Study the drawing (mm; zero at the part's minimum x, y, z) and answer. Coordinates: 2 decimals unless noted, no trailing zeros. Loops run counter-clockwise (first coordinate to the right, second up) from the corner with the lowest first, then second, coordinate; pieces in that order, holes last. Notation, with made-up numbers: (51.5, -30.5) -> (69.5, -30.5) arc R22 ccw to (69.5, -4.5) -> close; hole circle Ø10 at (35.25, 76.5). An arc over 180 degrees is marked (long way). One line per question, with ' | ' between items.
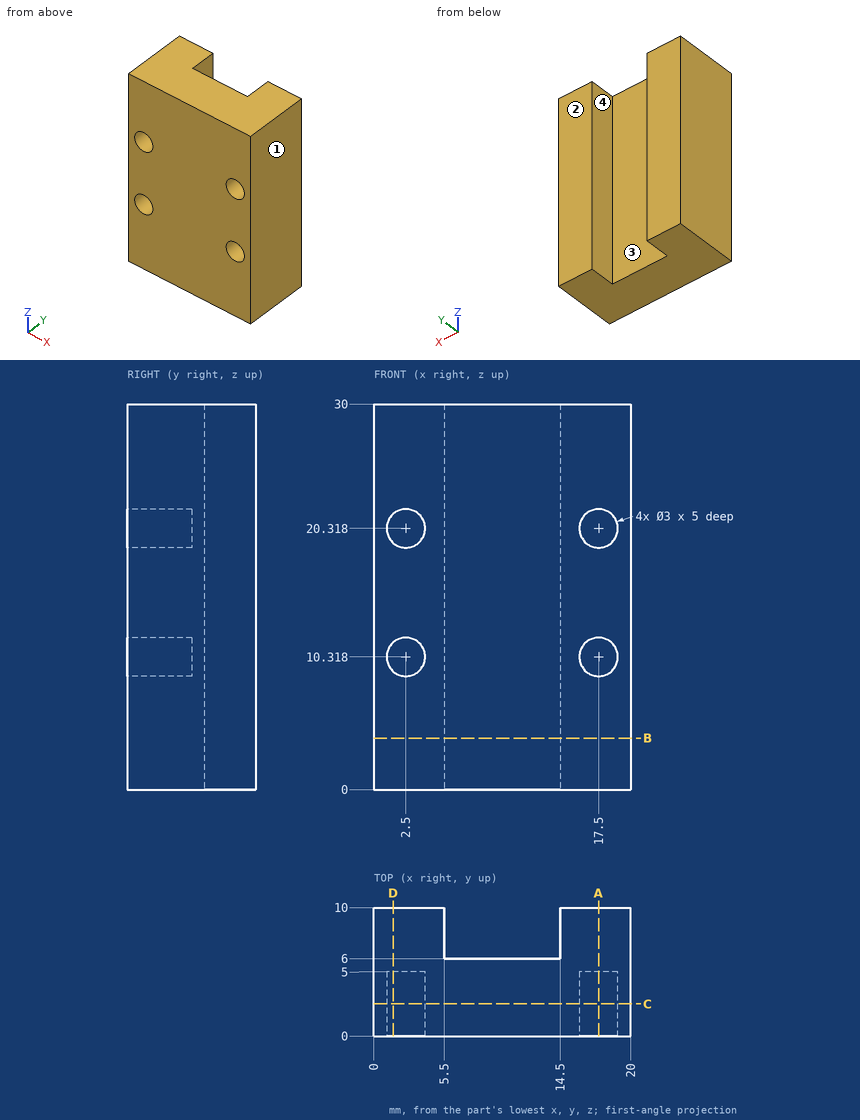
1) The mould has two halves that part along X. Classify the marked faces 1, 2, 3 and 4: released by +X, released by -X, zero draft, split by the parting line, or undercut.
Check values:
face 1: released by +X | face 2: zero draft | face 3: undercut | face 4: undercut
2) Find section D-D (x = 1.5). Write down the section's boundary in (y, z), plus the area to 3 significant figures.
Check values:
outline: (0, 0) -> (10, 0) -> (10, 30) -> (0, 30) -> (0, 21.44) -> (5, 21.44) -> (5, 19.2) -> (0, 19.2) -> (0, 11.44) -> (5, 11.44) -> (5, 9.2) -> (0, 9.2) -> close | area: 278 mm^2
3) Find section B-B (z = 4). Write down the section's boundary in (x, y).
Check values:
outline: (0, 0) -> (20, 0) -> (20, 10) -> (14.5, 10) -> (14.5, 6) -> (5.5, 6) -> (5.5, 10) -> (0, 10) -> close
4) Flat-ended cylindrical pins translate along their axes: pin 1 (1.5 mm diameter, centred on x = 12.5, z = 20, fed in from +Y); pin 2 (0.9 mm diameter, centred on x = 3, z = 20, fed in from -Y). Find the tip coordinate at first contact, or state that the pin passes through.
Check values:
pin 1: stops at y = 6 | pin 2: stops at y = 5
5) Find section A-A (x = 17.5). Write down the section's boundary in (y, z).
Check values:
outline: (0, 0) -> (10, 0) -> (10, 30) -> (0, 30) -> (0, 21.82) -> (5, 21.82) -> (5, 18.82) -> (0, 18.82) -> (0, 11.82) -> (5, 11.82) -> (5, 8.82) -> (0, 8.82) -> close
6) Find section C-C (y = 2.5). Write down the section's boundary in (x, z), plus the area to 3 significant figures.
Check values:
outline: (0, 0) -> (20, 0) -> (20, 30) -> (0, 30) -> close; hole circle Ø3 at (2.5, 10.32); hole circle Ø3 at (2.5, 20.32); hole circle Ø3 at (17.5, 10.32); hole circle Ø3 at (17.5, 20.32) | area: 572 mm^2
7) Find the intervals of material crossed by line 1 along Z through (x, y) = (17.5, 1.8); line 2 along X through (y, z) = (8.75, 26); line 3 along Z through (x, y) = (3.75, 4.25), in increasing order.
Check values:
line 1: z = 0 to 8.82, 11.82 to 18.82, 21.82 to 30 | line 2: x = 0 to 5.5, 14.5 to 20 | line 3: z = 0 to 9.49, 11.15 to 19.49, 21.15 to 30
